Model file for the job. Use its own axes, mm. A direction names the side the tool comes from. Round coordinates to 2 decimals unless told otherwise and drop trailing zeros. Loops run counter-clockwise (first coordinate to the right, second up) from the corner with the lowest first, then second, coordinate; pieces in that order, holes last. Notation, with made-up numbers: M 33,38 L 52,38 A3 ccw 52,42 Z; hole C 67,52.5 d11. An arc over 180 degrees is marked long. Use a Markdown table: item, result. Add a question column.
Item 1: Saw through at A-A on z = 78.5. Give the number of separate pieces and of enclosed holes in the cut face, then the cut area to 3 significant figures.
Item 2: Wall check: L1, parallel to Y at x = -208.5, z = 101 (3 decimals); L2, parallel to Y at x = -217, z = 31 (3 decimals); L3, parallel to X at y = -265, z = 1. Give the ranges that are in metal, low to high. Write a range as from..to.
Item 3: Saw through at D-D on x = -448. Write the cut outline in (y, z) (3 decimals), then the cut area to 4 significant figures.
Item 4: Saw through at C-C on y = -658.5. Write the cut outline in (x, z), then the cut area to 3 significant figures.
Item 5: Tool access for faces 1 (the flat face through (310, -528, 152.4)), 2 (the flat face through (-599, -409.575, 89)), 3 (the flat face through (-218, -257.175, 89)): list every direction of +Z, -Z, +X, -X, +Y, -Y with a clear straight run to the whole face (end or side of a thin tool).
Item 6: Saw through at B-B on x = 443.5. Write the cut outline in (y, z) (3 decimals).
Item 7: Pin check, flat tips, straight feed: P1, Ø5, axis at y = -473, z = 97, coming from the -X side; P2, Ø6, axis at x = 362.5, z = 123, coming from the +Y side (3 decimals); P3, Ø5, axis at y = -405.5, z = 122, coming from the +X side. Stop position of each tip, or through.
```python
from build123d import *

# Parameters (mm, degrees)
F0_W     = 1600.2
F0_H     = 901.7
F1_DEPTH = 25.4
F2_R     = 177.8
F3_DEPTH = 14.3002
F4_W     = 355.5433
F4_H     = 6.35
F4_R     = 82.55
F5_DEPTH = 152.4
F6_R     = 82.55
F7_DEPTH = 152.4


with BuildPart() as f1:
    # F0 (on Top) → F1 (new body)
    with BuildSketch(Plane.XY):
        with Locations((0, -450.85)):
            Rectangle(F0_W, F0_H)
    extrude(amount=-F1_DEPTH)

    # F2 (on face) → F3 (join)
    with BuildSketch(Plane.XY):
        with Locations((-596.9, -406.4)):
            Circle(F2_R)
        with Locations((-215.9, -254)):
            Circle(F2_R)
        with Locations((215.9, -254)):
            Circle(F2_R)
        with Locations((596.9, -406.4)):
            Circle(F2_R)
    extrude(amount=F3_DEPTH)

    # F4 (on face) → F5 (join)
    with BuildSketch(Plane.XY.offset(14.3002)):
        with Locations((-596.9, -406.4)):
            Rectangle(F4_W, F4_H)
        with Locations((-215.9, -254)):
            Rectangle(F4_W, F4_H)
        with Locations((215.9, -254)):
            Rectangle(F4_W, F4_H)
        with Locations((596.9, -406.4)):
            Rectangle(F4_W, F4_H)
        with Locations((-596.9, -499.11)):
            Circle(F4_R)
        with Locations((-596.9, -313.69)):
            Circle(F4_R)
        with Locations((-215.9, -161.29)):
            Circle(F4_R)
        with Locations((-215.9, -346.71)):
            Circle(F4_R)
        with Locations((215.9, -346.71)):
            Circle(F4_R)
        with Locations((215.9, -161.29)):
            Circle(F4_R)
        with Locations((596.9, -313.69)):
            Circle(F4_R)
        with Locations((596.9, -499.11)):
            Circle(F4_R)
    extrude(amount=F5_DEPTH)

    # F6 (on face) → F7 (join)
    with BuildSketch(Plane.XY):
        with Locations((-311.15, -529.59)):
            Circle(F6_R)
        with Locations((-114.3, -529.59)):
            Circle(F6_R)
        with Locations((114.3, -529.59)):
            Circle(F6_R)
        with Locations((311.15, -529.59)):
            Circle(F6_R)
    extrude(amount=F7_DEPTH)


solid = f1.part
```
Entries:
| question | item | result |
|---|---|---|
| 1 | separate pieces | 16 |
| 1 | enclosed holes | 0 |
| 1 | area | 266,000 mm2 |
| 2 | L1 | -428.928..-264.492, -257.175..-250.825, -243.508..-79.072 |
| 2 | L2 | -429.253..-264.167, -257.175..-250.825, -243.833..-78.747 |
| 2 | L3 | -704.69..-489.11, -393.36..-38.44, 38.44..393.36, 489.11..704.69 |
| 3 | outline | M -901.7,-25.4 L 0,-25.4 L 0,0 L -309.232,0 L -309.232,14.3 L -403.225,14.3 L -403.225,166.7 L -409.575,166.7 L -409.575,14.3 L -503.568,14.3 L -503.568,0 L -901.7,0 Z |
| 3 | area | 26,650 mm2 |
| 4 | outline | M -800.1,-25.4 L 800.1,-25.4 L 800.1,0 L -800.1,0 Z |
| 4 | area | 40,600 mm2 |
| 5 | face 1 | +Z, -Y |
| 5 | face 2 | +Z, -X |
| 5 | face 3 | +Z |
| 6 | outline | M -901.7,-25.4 L 0,-25.4 L 0,0 L -316.504,0 L -316.504,14.3 L -403.225,14.3 L -403.225,166.7 L -409.575,166.7 L -409.575,14.3 L -496.296,14.3 L -496.296,0 L -901.7,0 Z |
| 7 | P1 | x = -676 |
| 7 | P2 | y = -250.825 |
| 7 | P3 | x = 774.67 |
